```python
from build123d import *

# Parameters (mm, degrees)
SKETCH1_R           = 32.75
SKETCH1_R_2         = 15.25
SKETCH1_R_3         = 4.25
BOSS_EXTRUDE1_DEPTH = 10
SKETCH1_4_R         = 4.25
CUT_EXTRUDE2_DEPTH  = 94.934159921
CUT_EXTRUDE3_START  = 4
SKETCH1_6_R         = 32.75
SKETCH1_6_R_2       = 4.25
SKETCH1_6_R_3       = 15.25
CUT_EXTRUDE3_DEPTH  = 90.934159921
CHAMFER1_SIZE       = 1
CHAMFER2_SIZE       = 0.5


with BuildPart() as part:
    # Sketch1 → Boss-Extrude1 (new body)
    # profile 1 of 9: a face of its own
    with BuildSketch(Plane(origin=(0, 0, 0), x_dir=(1, 0, 0), z_dir=(0, 1, 0))):
        with BuildLine():
            Line((-40, -80.42), (40, -80.42))
            ThreePointArc((40, -80.42), (45.303300859, -78.223300859), (47.5, -72.92))
            Line((47.5, -72.92), (47.5, 32.08))
            ThreePointArc((47.5, 32.08), (45.303300859, 37.383300859), (40, 39.58))
            Line((40, 39.58), (-40, 39.58))
            ThreePointArc((-40, 39.58), (-45.303300859, 37.383300859), (-47.5, 32.08))
            Line((-47.5, 32.08), (-47.5, -72.92))
            ThreePointArc((-47.5, -72.92), (-45.303300859, -78.223300859), (-40, -80.42))
        make_face()
        Circle(SKETCH1_R, mode=Mode.SUBTRACT)
        with Locations((0, -58.34)):
            Circle(SKETCH1_R_2, mode=Mode.SUBTRACT)
        with BuildLine():
            ThreePointArc((46, 32.08), (40, 38.08), (34, 32.08))
            Line((34, 32.08), (34, -72.92))
            ThreePointArc((34, -72.92), (40, -78.92), (46, -72.92))
            Line((46, -72.92), (46, 32.08))
        make_face(mode=Mode.SUBTRACT)
        with BuildLine():
            ThreePointArc((-34, 32.08), (-40, 38.08), (-46, 32.08))
            Line((-46, 32.08), (-46, -72.92))
            ThreePointArc((-46, -72.92), (-40, -78.92), (-34, -72.92))
            Line((-34, -72.92), (-34, 32.08))
        make_face(mode=Mode.SUBTRACT)
    # profile 2 of 9: a face of its own
    with BuildSketch(Plane(origin=(0, 0, 0), x_dir=(1, 0, 0), z_dir=(0, 1, 0))):
        Circle(SKETCH1_R)
        Circle(SKETCH1_R_3, mode=Mode.SUBTRACT)
    # profile 3 of 9: a face of its own
    with BuildSketch(Plane(origin=(0, 0, 0), x_dir=(1, 0, 0), z_dir=(0, 1, 0))):
        with Locations((0, -58.34)):
            Circle(SKETCH1_R_2)
        with Locations((0, -58.34)):
            Circle(SKETCH1_R_3, mode=Mode.SUBTRACT)
    # profile 4 of 9: a face of its own
    with BuildSketch(Plane(origin=(0, 0, 0), x_dir=(1, 0, 0), z_dir=(0, 1, 0))):
        with BuildLine():
            Line((-34, -72.92), (-34, 32.08))
            ThreePointArc((-34, 32.08), (-40, 38.08), (-46, 32.08))
            Line((-46, 32.08), (-46, -72.92))
            ThreePointArc((-46, -72.92), (-40, -78.92), (-34, -72.92))
        make_face()
        with BuildLine():
            ThreePointArc((-43.25, -72.92), (-40, -76.17), (-36.75, -72.92))
            Line((-36.75, -72.92), (-36.75, 32.08))
            ThreePointArc((-36.75, 32.08), (-40, 35.33), (-43.25, 32.08))
            Line((-43.25, 32.08), (-43.25, -72.92))
        make_face(mode=Mode.SUBTRACT)
    # profile 5 of 9: a face of its own
    with BuildSketch(Plane(origin=(0, 0, 0), x_dir=(1, 0, 0), z_dir=(0, 1, 0))):
        with BuildLine():
            Line((46, -72.92), (46, 32.08))
            ThreePointArc((46, 32.08), (40, 38.08), (34, 32.08))
            Line((34, 32.08), (34, -72.92))
            ThreePointArc((34, -72.92), (40, -78.92), (46, -72.92))
        make_face()
        with BuildLine():
            ThreePointArc((36.75, -72.92), (40, -76.17), (43.25, -72.92))
            Line((43.25, -72.92), (43.25, 32.08))
            ThreePointArc((43.25, 32.08), (40, 35.33), (36.75, 32.08))
            Line((36.75, 32.08), (36.75, -72.92))
        make_face(mode=Mode.SUBTRACT)
    # profile 6 of 9: a face of its own
    with BuildSketch(Plane(origin=(0, 0, 0), x_dir=(1, 0, 0), z_dir=(0, 1, 0))):
        with BuildLine():
            Line((36.75, 32.08), (36.75, -72.92))
            ThreePointArc((36.75, -72.92), (40, -76.17), (43.25, -72.92))
            Line((43.25, -72.92), (43.25, 32.08))
            ThreePointArc((43.25, 32.08), (40, 35.33), (36.75, 32.08))
        make_face()
    # profile 7 of 9: a face of its own
    with BuildSketch(Plane(origin=(0, 0, 0), x_dir=(1, 0, 0), z_dir=(0, 1, 0))):
        with BuildLine():
            Line((-43.25, 32.08), (-43.25, -72.92))
            ThreePointArc((-43.25, -72.92), (-40, -76.17), (-36.75, -72.92))
            Line((-36.75, -72.92), (-36.75, 32.08))
            ThreePointArc((-36.75, 32.08), (-40, 35.33), (-43.25, 32.08))
        make_face()
    # profile 8 of 9: a face of its own
    with BuildSketch(Plane(origin=(0, 0, 0), x_dir=(1, 0, 0), z_dir=(0, 1, 0))):
        Circle(SKETCH1_R_3)
    # profile 9 of 9: a face of its own
    with BuildSketch(Plane(origin=(0, 0, 0), x_dir=(1, 0, 0), z_dir=(0, 1, 0))):
        with Locations((0, -58.34)):
            Circle(SKETCH1_R_3)
    extrude(amount=BOSS_EXTRUDE1_DEPTH)

    # Sketch1<4> → Cut-Extrude2 (cut, through all)
    with BuildSketch(Plane(origin=(0, 0, 0), x_dir=(1, 0, 0), z_dir=(0, 1, 0))):
        with BuildLine():
            Line((36.75, 32.08), (36.75, -72.92))
            ThreePointArc((36.75, -72.92), (40, -76.17), (43.25, -72.92))
            Line((43.25, -72.92), (43.25, 32.08))
            ThreePointArc((43.25, 32.08), (40, 35.33), (36.75, 32.08))
        make_face()
        with Locations(Location((0, 0, 0), (0, 0, 270))):
            Circle(SKETCH1_4_R)
        with Locations(Location((0, -58.34, 0), (0, 0, 270))):
            Circle(SKETCH1_4_R)
        with BuildLine():
            Line((-43.25, 32.08), (-43.25, -72.92))
            ThreePointArc((-43.25, -72.92), (-40, -76.17), (-36.75, -72.92))
            Line((-36.75, -72.92), (-36.75, 32.08))
            ThreePointArc((-36.75, 32.08), (-40, 35.33), (-43.25, 32.08))
        make_face()
    extrude(amount=CUT_EXTRUDE2_DEPTH, mode=Mode.SUBTRACT)

    # Sketch1<6> → Cut-Extrude3 (cut, through all)
    # profile 1 of 2: a face of its own
    with BuildSketch(Plane(origin=(0, 0, 0), x_dir=(1, 0, 0), z_dir=(0, 1, 0)).offset(CUT_EXTRUDE3_START)):
        with Locations(Location((0, 0, 0), (0, 0, 270))):
            Circle(SKETCH1_6_R)
        with Locations(Location((0, 0, 0), (0, 0, 270))):
            Circle(SKETCH1_6_R_2, mode=Mode.SUBTRACT)
    # profile 2 of 2: a face of its own
    with BuildSketch(Plane(origin=(0, 0, 0), x_dir=(1, 0, 0), z_dir=(0, 1, 0)).offset(CUT_EXTRUDE3_START)):
        with Locations(Location((0, -58.34, 0), (0, 0, 270))):
            Circle(SKETCH1_6_R_3)
        with Locations(Location((0, -58.34, 0), (0, 0, 270))):
            Circle(SKETCH1_6_R_2, mode=Mode.SUBTRACT)
    extrude(amount=CUT_EXTRUDE3_DEPTH, mode=Mode.SUBTRACT)

    # Chamfer1
    chamfer1_edges = [part.edges().sort_by_distance(p)[0] for p in [
        (0, 10, -32.75),
        (0, 10, 43.09),
    ]]
    chamfer(chamfer1_edges, length=CHAMFER1_SIZE)

    # Chamfer2
    chamfer2_edges = [part.edges().sort_by_distance(p)[0] for p in [
        (45.303300859, 10, 78.223300859),
        (-47.5, 0, 20.42),
        (-45.303300859, 0, -37.383300859),
        (0, 0, -39.58),
        (45.303300859, 0, -37.383300859),
        (47.5, 0, 20.42),
        (45.303300859, 0, 78.223300859),
        (0, 0, 80.42),
        (47.5, 10, 20.42),
        (45.303300859, 10, -37.383300859),
        (0, 10, -39.58),
        (-45.303300859, 10, -37.383300859),
        (-47.5, 10, 20.42),
        (36.75, 0, 20.42),
        (40, 0, 76.17),
        (43.25, 10, 20.42),
        (40, 0, -35.33),
        (36.75, 10, 20.42),
        (-45.303300859, 10, 78.223300859),
        (40, 10, 76.17),
        (40, 10, -35.33),
        (43.25, 0, 20.42),
        (0, 0, -4.25),
        (0, 0, 54.09),
        (-43.25, 0, 20.42),
        (-40, 0, 76.17),
        (-36.75, 10, 20.42),
        (-40, 0, -35.33),
        (-43.25, 10, 20.42),
        (-40, 10, 76.17),
        (-40, 10, -35.33),
        (0, 10, 80.42),
        (-36.75, 0, 20.42),
        (0, 4, -4.25),
        (0, 4, 54.09),
        (-45.303300859, 0, 78.223300859),
    ]]
    chamfer(chamfer2_edges, length=CHAMFER2_SIZE)


solid = part.part
```
Input: part model. Units: mm. Frame: model coordinates. A direction names the side the tool comes from. Coordinates: 2 decimals unless noted, no trailing zeros. Loops run counter-clockwise (first coordinate to the right, second up) from the corner with the lowest first, then second, coordinate; pieces in that order, holes last. Notation, with made-up numbers: M -10.5,20.25 L 29.5,20.25 A18 ccw 29.5,53.25 Z; hole C 57.25,14 d10. An arc over 180 degrees is marked long. Answer in a Markdown table with one row per item.
1. First-contact query: pin 1 (6 mm diameter, centred on x = 14, z = 4.5, fed in from +Y). Flat tip, straight axial feed; report the tip coordinate or a pass-through.
Response:
| item | result |
|---|---|
| pin 1 | stops at y = 4 |
2. Draft query along X for faces 6 (the cylindrical face through (-45.361, 4.937, 78.165)), 7 (the flat face through (1, 5, -39.58)), 8 (the flat face through (36.75, 5, 20)), 9 (the flat face through (47.5, 5, 21)). Return one class per face: pulls with the +X half, pulls with the -X half, needs draft (parallel to the pull), parting line crosses it, or undercut.
Response:
| item | result |
|---|---|
| face 6 | pulls with the -X half |
| face 7 | needs draft |
| face 8 | undercut |
| face 9 | pulls with the +X half |
3. Reachability of faces 1 (the cylindrical face through (45.245, 4.937, 78.281)), 2 (the conical face through (39.93, 0.36, 76.31)), 3 (the flat face through (-36.75, 5, 21)), 4 (the conical face through (-45.11, 9.86, 77.91)), 5 (the conical face through (-40.074, 9.635, -35.465)) from +Z, -Z, +X, -X, +Y, -Y: full face, straight path, thin tool, end or side. Return the list, or none.
Response:
| item | result |
|---|---|
| face 1 | +Z, +X, +Y, -Y |
| face 2 | -Y |
| face 3 | +Y, -Y |
| face 4 | +Z, -X, +Y |
| face 5 | +Y |
4. Section A-A, the plane z = 38. Output: boundary loops of the cut face in (x, y), then the cut area to 4 significant figures.
Response:
| item | result |
|---|---|
| outline | M -47.5,0.5 L -47,0 L -43.75,0 L -43.25,0.5 L -43.25,9.5 L -43.75,10 L -47,10 L -47.5,9.5 Z; M -36.75,0.5 L -36.25,0 L 36.25,0 L 36.75,0.5 L 36.75,9.5 L 36.25,10 L -36.25,10 L -36.75,9.5 Z; M 43.25,0.5 L 43.75,0 L 47,0 L 47.5,0.5 L 47.5,9.5 L 47,10 L 43.75,10 L 43.25,9.5 Z |
| area | 818.5 mm2 |
5. Material intervals for line 1 (Z direction, x = 0, y = 6.75); line 2 (X direction, y = 1.75, z = 33.5); line 3 (X direction, y = 7.7, z = 0), sorted ascending.
Response:
| item | result |
|---|---|
| line 1 | z = -39.58 to -32.75, 32.75 to 43.09, 73.59 to 80.42 |
| line 2 | x = -47.5 to -43.25, -36.75 to 36.75, 43.25 to 47.5 |
| line 3 | x = -47.5 to -43.25, -36.75 to -32.75, 32.75 to 36.75, 43.25 to 47.5 |
6. Section B-B, the plane y = 1.75. Output: boundary loops of the cut face in (x, z).
Response:
| item | result |
|---|---|
| outline | M -47.5,-32.08 A7.5 ccw -40,-39.58 L 40,-39.58 A7.5 ccw 47.5,-32.08 L 47.5,72.92 A7.5 ccw 40,80.42 L -40,80.42 A7.5 ccw -47.5,72.92 Z; hole M -43.25,-32.08 A3.25 ccw -36.75,-32.08 L -36.75,72.92 A3.25 ccw -43.25,72.92 Z; hole C 0,0 d8.5; hole C 0,58.34 d8.5; hole M 36.75,-32.08 A3.25 ccw 43.25,-32.08 L 43.25,72.92 A3.25 ccw 36.75,72.92 Z |
7. Section C-C, the plane z = 0. Count the separate pieces of the cut face and the enclosed holes in it, then the cut area to 3 significant figures.
Response:
| item | result |
|---|---|
| separate pieces | 4 |
| enclosed holes | 0 |
| area | 390 mm2 |
